```python
from build123d import *

# Parameters (mm, degrees)
SKETCH1_W           = 17.3609
SKETCH1_H           = 12.7
BOSS_EXTRUDE1_DEPTH = 13.97
SKETCH2_W           = 20.828
SKETCH2_H           = 14.9352
BOSS_EXTRUDE2_DEPTH = 2.032
SKETCH3_W           = 4.7752
SKETCH3_H           = 0.8382
BOSS_EXTRUDE3_DEPTH = 8.0772
FILLET1_RADIUS      = 2.3876
FILLET1_LENGTH      = 0.8382
FILLET2_RADIUS      = 2.3876
FILLET2_LENGTH      = 0.8382


with BuildPart() as part:
    # Sketch1 → Boss-Extrude1 (new body)
    with BuildSketch(Plane(origin=(0, 0, 0), x_dir=(1, 0, 0), z_dir=(0, 1, 0))):
        with Locations((8.68045, 6.35)):
            Rectangle(SKETCH1_W, SKETCH1_H)
    extrude(amount=-BOSS_EXTRUDE1_DEPTH)

    # Sketch2 → Boss-Extrude2 (add)
    with BuildSketch(Plane(origin=(0, 0, 0), x_dir=(1, 0, 0), z_dir=(0, 1, 0))):
        with Locations((8.68045, 6.35)):
            Rectangle(SKETCH2_W, SKETCH2_H)
    extrude(amount=BOSS_EXTRUDE2_DEPTH)

    # Sketch3 → Boss-Extrude3 (add)
    with BuildSketch(Plane.XZ.offset(13.97)):
        with Locations((4.9276, -2.3241)):
            Rectangle(SKETCH3_W, SKETCH3_H)
        with Locations((13.1953, -3.7592)):
            Rectangle(SKETCH3_W, SKETCH3_H)
    extrude(amount=BOSS_EXTRUDE3_DEPTH)

    # Fillet1: full round fillet: the end face becomes a half cylinder, R = half its width
    fillet1_face = Plane((4.9276, -22.0472, -2.3241), x_dir=(0, 0, -1), z_dir=(0, -1, 0))  # on the end face: x along it, z out of the body
    fillet1_slab = fillet1_face.offset(-FILLET1_RADIUS / 2) * Box(FILLET1_LENGTH, 2 * FILLET1_RADIUS, FILLET1_RADIUS, mode=Mode.PRIVATE)  # the body's end, R deep
    fillet1_round = Plane((4.9276, -19.6596, -2.3241), x_dir=(0, -1, 0), z_dir=(0, 0, -1)) * Cylinder(FILLET1_RADIUS, FILLET1_LENGTH, mode=Mode.PRIVATE)  # its axis R under the face
    add(fillet1_slab - fillet1_round, mode=Mode.SUBTRACT)

    # Fillet2: full round fillet: the end face becomes a half cylinder, R = half its width
    fillet2_face = Plane((13.1953, -22.0472, -3.7592), x_dir=(0, 0, -1), z_dir=(0, -1, 0))  # on the end face: x along it, z out of the body
    fillet2_slab = fillet2_face.offset(-FILLET2_RADIUS / 2) * Box(FILLET2_LENGTH, 2 * FILLET2_RADIUS, FILLET2_RADIUS, mode=Mode.PRIVATE)  # the body's end, R deep
    fillet2_round = Plane((13.1953, -19.6596, -3.7592), x_dir=(0, -1, 0), z_dir=(0, 0, -1)) * Cylinder(FILLET2_RADIUS, FILLET2_LENGTH, mode=Mode.PRIVATE)  # its axis R under the face
    add(fillet2_slab - fillet2_round, mode=Mode.SUBTRACT)


solid = part.part
```
For this review, take the finished solid that the model builds, in its own axes (mm). A direction names the side the tool comes from. Round coordinates to 2 decimals unless told otherwise and drop trailing zeros. Write each loop counter-clockwise with the first axis right and the second up, starting at its lowest first coordinate (ties: lowest second). Pieces come first, ordered by that corner, then holes. Notation, with made-up numbers: (23, 66.25) - (65, 66.25) arc R15 cw to (65, 86.25) - close; hole circle Ø3 at (4, 54.25). An arc over 180 degrees is marked (long way). Use CSV: the item, a comma, the result in double quotes.
1) Add section C-C on x = 1. Write out the cut boundary in (y, z).
Conclusion:
outline,"(-13.97, -12.7) - (0, -12.7) - (0, -13.82) - (2.03, -13.82) - (2.03, 1.12) - (0, 1.12) - (0, 0) - (-13.97, 0) - close"
2) Add section D-D on y = -20.25. Write out the cut boundary in (x, z) (3 decimals).
Conclusion:
outline,"(2.614, -2.743) - (7.241, -2.743) - (7.241, -1.905) - (2.614, -1.905) - close; (10.882, -4.178) - (15.509, -4.178) - (15.509, -3.34) - (10.882, -3.34) - close"
3) Clearance check with flat-ended pins moving along their axes: pin 1 Ø2 at (x, z) = (16.5, -6.5) entering from -Y; pin 2 Ø0.7 at (y, z) = (-18, -2.5) entering from +X; pin 3 Ø4 at (y, z) = (-8.5, -3.5) entering from -X; pin 4 Ø1 at (y, z) = (-16, -9.5) entering from -X. State where each tip first meets the part, or that it passes through.
Conclusion:
pin 1,"stops at y = -13.97"
pin 2,"stops at x = 7.32"
pin 3,"stops at x = 0"
pin 4,"passes through"
4) For faces 1 (the flat face through (5, -18, -1.905)), 2 (the flat face through (7.315, -16.8, -2.3)), 3 (the flat face through (13, -18, -4.178)), list the 3-axis set-ups (+Z, -Z, +X, -X, +Y, -Y) from which the entire face can be reached by the end or side of a thin tool; tool diameter is ignored.
Conclusion:
face 1,"+Z, +X, -X, -Y"
face 2,"+Z, -Z, +X, -Y"
face 3,"-Z, +X, -X, -Y"
5) The part is to be moulded in two halves that separate along Z. For faces 4 (the flat face through (19.094, 1, -6)), 5 (the flat face through (5, -18, -2.743)), 6 (the flat face through (9, -7, 0)), say which applies: pulls with the +Z half, pulls with the -Z half, needs draft (parallel to the pull), parting line crosses it, or undercut.
Conclusion:
face 4,"needs draft"
face 5,"pulls with the -Z half"
face 6,"pulls with the +Z half"
6) Wall thickness on line 1 along X through (y, z) = (-11, -1); line 2 along Z through (x, y) = (12.5, -17); line 3 along Y through (x, z) = (4.75, -11.25): over which ranges is each line inside the solid? List them lowest first. Write a range as from..to.
Conclusion:
line 1,"x = 0..17.36"
line 2,"z = -4.18..-3.34"
line 3,"y = -13.97..2.03"
7) Add section A-A on y = -15. Write out the cut boundary in (x, z) (3 decimals), and give its area (3 significant figures).
Conclusion:
outline,"(2.54, -2.743) - (7.315, -2.743) - (7.315, -1.905) - (2.54, -1.905) - close; (10.808, -4.178) - (15.583, -4.178) - (15.583, -3.34) - (10.808, -3.34) - close"
area,"8.01 mm^2"
8) Add section B-B on z = -8.5. Write out the cut boundary in (x, y).
Conclusion:
outline,"(-1.73, 0) - (0, 0) - (0, -13.97) - (17.36, -13.97) - (17.36, 0) - (19.09, 0) - (19.09, 2.03) - (-1.73, 2.03) - close"
